Geometry check sheet. Reference: drawing and pictorial views, mm from the part's lowest x, y, z. Coordinates: 2 decimals unless noted, no trailing zeros. Order: outer loops, then holes, each group sorted by start corner. A loop starts at its lowest first (then second) coordinate and runs counter-clockwise, first axis right, second up. Notation, with made-up numbers: (-5.5, 50) -> (18.5, 50) arc R23 ccw to (18.5, 84) -> close; hole circle Ø1 at (46, 76.5). An arc over 180 degrees is marked (long way). Use CSV: the item, a comma, the result in double quotes. Start each with the question number.
1) Sectioned sample at C-C on y = 222. Record the boundary of the cut face in (x, z), then the cut area to 3 significant figures.
2) Go/stop test with a flat-tipped pin: pin 1 (2 mm diameter, centred on y = 70, z = 1.5, fed in from +X). Record where the tip stops, or that it passes through.
3) Scan lines: line 1 along Y through (x, z) = (270.5, 3.7) (1 decimal); line 2 along X through (y, z) = (43, 1.8) (1 decimal); line 3 along Y through (x, z) = (306, 2.85) (1 decimal). Record each from-to range of solid material in increasing order.
4) Sectioned sample at A-A on x = 281. Record the boundary of the cut face in (y, z), then the cut area to 3 significant figures.
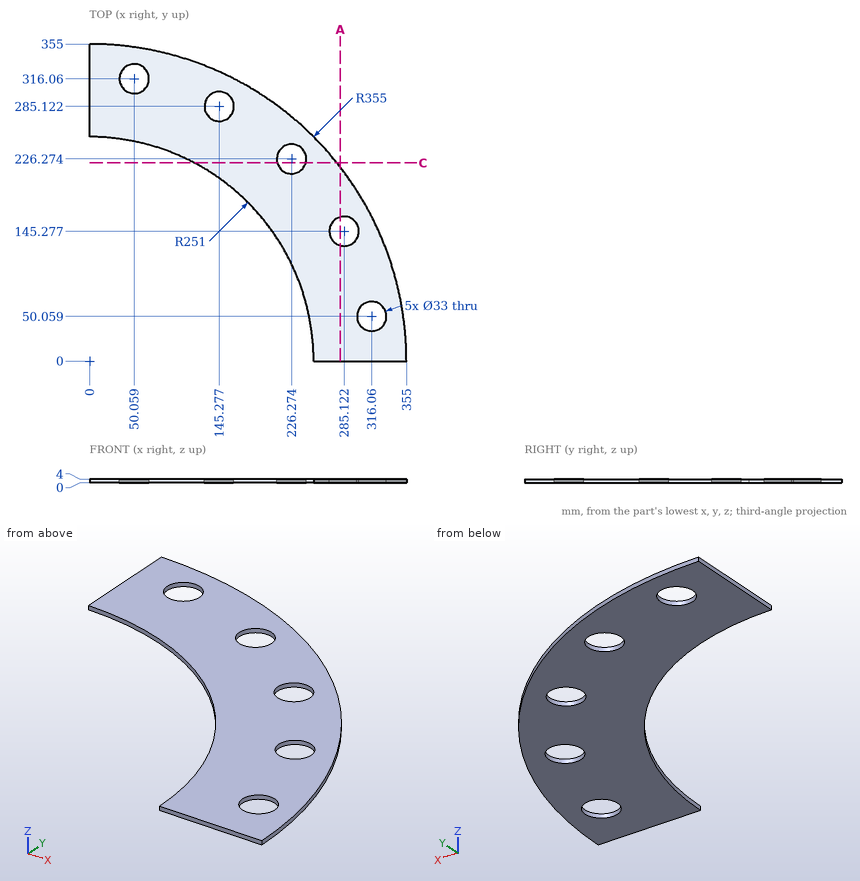
Answers follow:
1,outline,"(117.12, 0) -> (210.34, 0) -> (210.34, 4) -> (117.12, 4) -> close; (242.21, 0) -> (277.02, 0) -> (277.02, 4) -> (242.21, 4) -> close"
1,area,"512 mm²"
2,pin 1,"stops at x = 348.23"
3,line 1,"y = 0 to 137.6, 152.9 to 229.9"
3,line 2,"x = 247.3 to 301.1, 331 to 352.4"
3,line 3,"y = 0 to 37, 63.1 to 180"
4,outline,"(0, 0) -> (129.3, 0) -> (129.3, 4) -> (0, 4) -> close; (161.25, 0) -> (216.94, 0) -> (216.94, 4) -> (161.25, 4) -> close"
4,area,"740 mm²"
